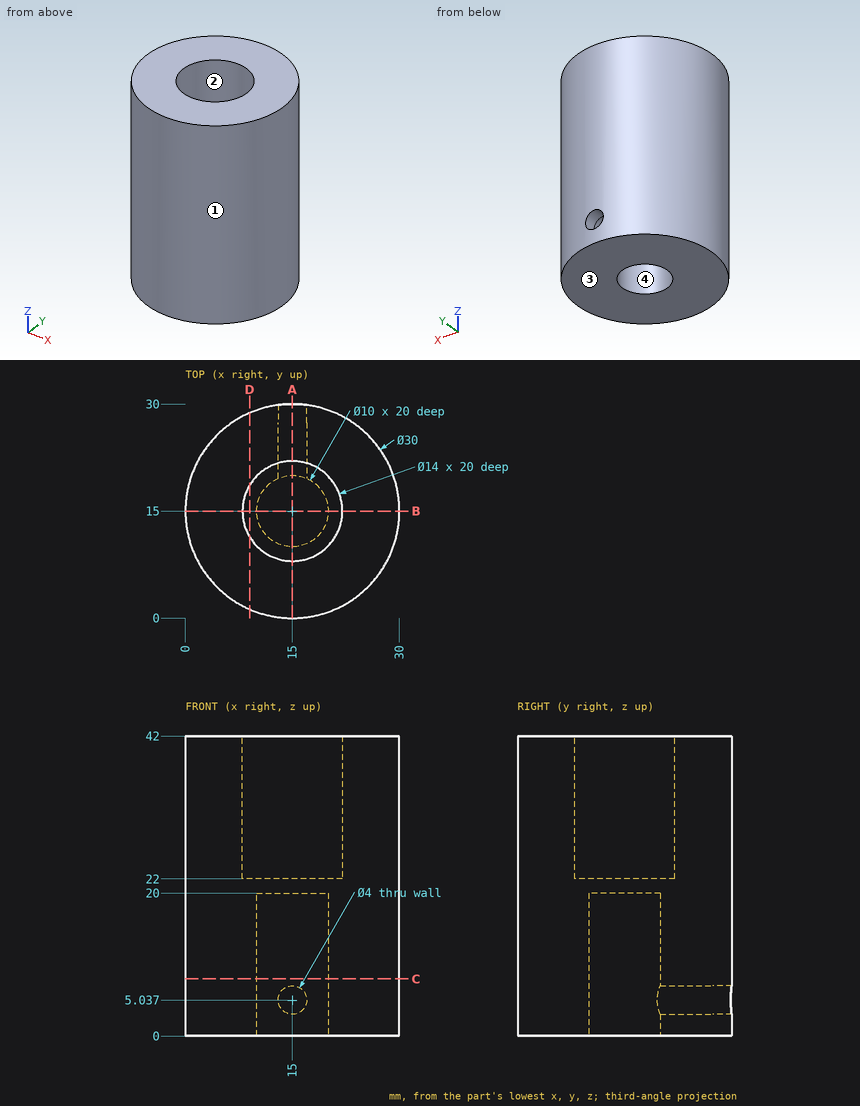
Part print with two shaded views. Sizes in mm from the minimum x, y, z corner. Coordinates: 2 decimals unless noted, no trailing zeros. Write each loop counter-clockwise with the first axis right and the second up, starting at its lowest first coordinate (ties: lowest second). Pieces come first, ordered by that corner, then holes. Notation, with made-up numbers: (11.25, 32.5) -> (61.25, 32.5) arc R27 cw to (61.25, 49.5) -> close; hole circle Ø5 at (-4.5, 34). An arc over 180 degrees is marked (long way). Return JSON: item names as keys, results as strings. Group by question number.
Q1. Cut at C-C, the plane z = 8. Give the cut face in (x, y), then the cut area to 3 significant figures.
Q2. Cut at A-A, the plane x = 15. Give the cut face in (y, z), then the cut area to 3 significant figures.
Q3. Flat gauge pins, fed straight in: pin 1 (4 mm diameter, centred on x = 14.5, y = 18, fed in from +Z); pin 2 (2 mm diameter, centred on y = 10.5, z = 23.5, fed in from -X); pin 3 (6 mm diameter, centred on y = 18.5, z = 11, fed in from +X). Where does each tip first touch, or does it go through?
Q4. Pull direction Y, two halves, no side cores. Call the marked faces 1, 2, 3 and 4: released by +Y, released by -Y, zero draft, split by the parting line, or undercut.
Q5. Drill centre lines: line 1 (Y direction, x = 15, z = 14); line 2 (Z direction, x = 15, y = 28.8); line 3 (Y direction, x = 15, z = 36). Where is each one in solid material? Low to high.
Q6. Cut at B-B, the plane y = 15. Give the cut face in (x, z), then the cut area to 3 significant figures.
Q7. Cut at D-D, the plane x = 9. Give the cut face in (y, z).
Returned:
{
 "1": {"outline": "circle Ø30 at (15, 15); hole circle Ø10 at (15, 15)", "area": "628 mm2"},
 "2": {"outline": "(0, 0) -> (10, 0) -> (10, 20) -> (20, 20) -> (20, 7.04) -> (30, 7.04) -> (30, 42) -> (22, 42) -> (22, 22) -> (8, 22) -> (8, 42) -> (0, 42) -> close; (20, 0) -> (30, 0) -> (30, 3.04) -> (20, 3.04) -> close", "area": "740 mm2"},
 "3": {"pin 1": "stops at z = 22", "pin 2": "stops at x = 0.41", "pin 3": "stops at x = 29.99"},
 "4": {"face 1": "split by the parting line", "face 2": "undercut", "face 3": "zero draft", "face 4": "undercut"},
 "5": {"line 1": "y = 0 to 10, 20 to 30", "line 2": "z = 0 to 3.04, 7.04 to 42", "line 3": "y = 0 to 8, 22 to 30"},
 "6": {"outline": "(0, 0) -> (10, 0) -> (10, 20) -> (20, 20) -> (20, 0) -> (30, 0) -> (30, 42) -> (22, 42) -> (22, 22) -> (8, 22) -> (8, 42) -> (0, 42) -> close", "area": "780 mm2"},
 "7": {"outline": "(1.25, 0) -> (28.75, 0) -> (28.75, 42) -> (18.61, 42) -> (18.61, 22) -> (11.39, 22) -> (11.39, 42) -> (1.25, 42) -> close"}
}
